Input: part model. Units: mm. Frame: model coordinates. Face numbers are marked on the shaded views. A direction names the side the tool comes from. Coordinates: 2 decimals unless noted, no trailing zeros. Write each loop counter-clockwise with the first axis right and the second up, starting at its lowest first coordinate (ties: lowest second). Pieces come first, ordered by that corner, then holes. Notation, with made-up numbers: M 39,-37.5 L 46,-37.5 A23 ccw 46,-25.5 Z; hole C 75,-25 d1. An arc over 180 degrees is marked long. Use one line per item in the form item = value.
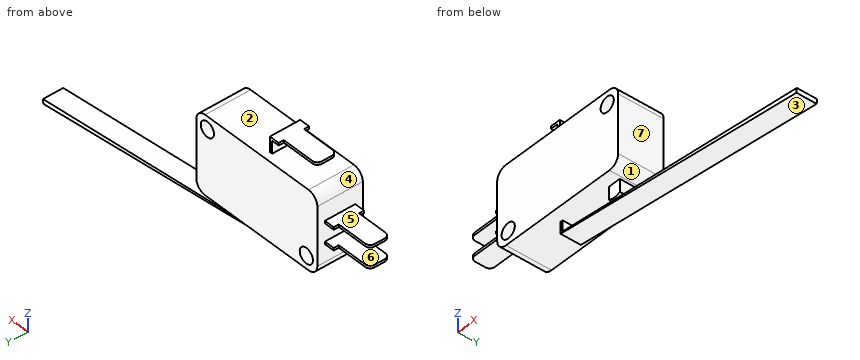
from build123d import *

# Parameters (mm, degrees)
SKETCH1_R            = 1.5
BOSS_EXTRUDE1_DEPTH  = 9
BOSS_EXTRUDE2_DEPTH  = 4
BOSS_EXTRUDE9_DEPTH  = 4
SKETCH5_W            = 9
SKETCH5_H            = 0.5
BOSS_EXTRUDE10_DEPTH = 6
SKETCH6_W            = 7.5
SKETCH6_H            = 1
CUT_EXTRUDE1_DEPTH   = 2
SKETCH7_W            = 7
SKETCH7_H            = 1
CUT_EXTRUDE2_DEPTH   = 5
FILLET1_R            = 1


with BuildPart() as part:
    # Sketch1 → Boss-Extrude1 (new body)
    with BuildSketch(Plane(origin=(0, 0, 0), x_dir=(1, 0, 0), z_dir=(0, 1, 0))):
        with BuildLine():
            Line((11.75, -7.75), (-11.75, -7.75))
            ThreePointArc((-11.75, -7.75), (-13.164213562, -7.164213562), (-13.75, -5.75))
            Line((-13.75, -5.75), (-13.75, 5.75))
            ThreePointArc((-13.75, 5.75), (-13.164213562, 7.164213562), (-11.75, 7.75))
            Line((-11.75, 7.75), (11.75, 7.75))
            ThreePointArc((11.75, 7.75), (13.164213562, 7.164213562), (13.75, 5.75))
            Line((13.75, 5.75), (13.75, -5.75))
            ThreePointArc((13.75, -5.75), (13.164213562, -7.164213562), (11.75, -7.75))
        make_face()
        with Locations(Location((-11.25, 5.25, 0), (0, 0, 270))):
            Circle(SKETCH1_R, mode=Mode.SUBTRACT)
        with Locations(Location((11.25, -5.25, 0), (0, 0, 270))):
            Circle(SKETCH1_R, mode=Mode.SUBTRACT)
    extrude(amount=BOSS_EXTRUDE1_DEPTH)

    # Sketch3 → Boss-Extrude2 (add)
    with BuildSketch(Plane(origin=(0, 2.5, 0), x_dir=(-1, 0, 0), z_dir=(0, -1, 0))):
        with BuildLine():
            Line((-11.25, 7.75), (-11.25, 10.25))
            ThreePointArc((-11.25, 10.25), (-10, 10.584936491), (-8.75, 10.25))
            Line((-8.75, 10.25), (-8.75, 7.75))
            Line((-8.75, 7.75), (-11.25, 7.75))
        make_face()
    extrude(amount=-BOSS_EXTRUDE2_DEPTH)

    # Sketch4 → Boss-Extrude9 (add)
    with BuildSketch(Plane(origin=(0, 2.5, 0), x_dir=(-1, 0, 0), z_dir=(0, -1, 0))):
        Polygon((1.75, 7.75), (2.205022523, 7.75), (2.205022523, 10.069490078), (-51.392713573, 15.829296812), (-51.47623297, 14.95318025), (1.75, 9.879171754), align=None)
    extrude(amount=-BOSS_EXTRUDE9_DEPTH)

    # Sketch5 → Boss-Extrude10 (add)
    with BuildSketch(Plane(origin=(0, 1.5, 0), x_dir=(-1, 0, 0), z_dir=(0, -1, 0))):
        Polygon((1.75, -7.75), (1.75, -10.25), (10.75, -10.25), (10.75, -10.75), (1.25, -10.75), (1.25, -7.75), align=None)
        with Locations((18.25, 2.049029433)):
            Rectangle(SKETCH5_W, SKETCH5_H)
        with Locations((18.25, -1.950970567)):
            Rectangle(SKETCH5_W, SKETCH5_H)
    extrude(amount=-BOSS_EXTRUDE10_DEPTH)

    # Sketch6 → Cut-Extrude1 (cut)
    with BuildSketch(Plane.XY.offset(10.75)):
        with Locations((-7, 2)):
            Rectangle(SKETCH6_W, SKETCH6_H)
        with Locations((-7, 7)):
            Rectangle(SKETCH6_W, SKETCH6_H)
    extrude(amount=-CUT_EXTRUDE1_DEPTH, mode=Mode.SUBTRACT)

    # Sketch7 → Cut-Extrude2 (cut)
    with BuildSketch(Plane.XY.offset(2.200970567)):
        with Locations((-19.25, 2)):
            Rectangle(SKETCH7_W, SKETCH7_H)
        with Locations((-19.25, 7)):
            Rectangle(SKETCH7_W, SKETCH7_H)
    extrude(amount=-CUT_EXTRUDE2_DEPTH, mode=Mode.SUBTRACT)

    # Fillet1
    fillet1_edges = [part.edges().sort_by_distance(p)[0] for p in [
        (-10.75, 2.5, 10.5),
        (-10.75, 6.5, 10.5),
        (-22.75, 2.5, -2.049029433),
        (-22.75, 2.5, 1.950970567),
        (-22.75, 6.5, -2.049029433),
        (-22.75, 6.5, 1.950970567),
    ]]
    fillet(fillet1_edges, radius=FILLET1_R)


solid = part.part
(1) Line query: probe 1 along X at (y, z) = (7, -5.25); probe 2 along X at (y, z) = (2.75, 5.25); probe 3 along X at (y, z) = (2, 0.5). Output: solid intervals per line, ascending.
Computed:
probe_1 = -13.75 to -12.75, -9.75 to 13.75
probe_2 = -13.75 to 9.75, 12.75 to 13.75
probe_3 = -13.75 to 13.75
(2) Section query A-A on x = -14.5. Return the cut outline in (y, z), plus the area to 3 significant figures.
Computed:
outline = M 1.5,-2.3 L 7.5,-2.3 L 7.5,-1.8 L 1.5,-1.8 Z; M 1.5,1.7 L 7.5,1.7 L 7.5,2.2 L 1.5,2.2 Z
area = 6.00 mm^2
(3) Section query C-C on z = 0.5. Return the cut outline in (x, y).
Computed:
outline = M -13.75,0 L 13.75,0 L 13.75,9 L -13.75,9 Z
(4) Set-up query: the marked faces 5, 6 and 7. Return all of +Z, -Z, +X, -X, +Y, -Y with unobstructed straight access to the full face (end or side cutting, diameter ignored); none if empty.
Computed:
face_5 = +Z, -X, +Y, -Y
face_6 = -X, +Y, -Y
face_7 = +Z, +X, +Y, -Y
(5) First-contact query: pin 1 Ø2 at (y, z) = (7.5, 1.5) entering from +X; pin 2 Ø3 at (x, y) = (-16.5, 5) entering from -Z; pin 3 Ø1.5 at (x, y) = (11.5, 5) entering from +Z; pin 4 Ø2.5 at (x, z) = (-11.25, -5.25) entering from +Y. Flat tips, straight axial feed; report the tip coordinate or a pass-through.
Computed:
pin_1 = 13.75
pin_2 = -2.3
pin_3 = 7.75
pin_4 = through
(6) Section query D-D on x = 0.5. Return the cut outline in (y, z).
Computed:
outline = M 0,-7.75 L 9,-7.75 L 9,7.75 L 0,7.75 Z; M 2.5,-10.36 L 6.5,-10.36 L 6.5,-10.09 L 2.5,-10.09 Z
(7) Section query B-B on y = 4.75. State how many separate pieces and enclosed holes the cut face has, plus the area to 3 significant figures.
Computed:
separate_pieces = 1
enclosed_holes = 2
area = 461 mm^2
(8) Pull-direction query (Z, two-part tool) for the marked faces 1, 2, 3 and 4; classes: pulls with the +Z half, pulls with the -Z half, needs draft (parallel to the pull), parting line crosses it, or undercut.
Computed:
face_1 = undercut
face_2 = undercut
face_3 = pulls with the -Z half
face_4 = pulls with the +Z half
